```python
from build123d import *

# Parameters (mm, degrees)
ESQUISSE1_R        = 1.5
BOSS_EXTRU_2_DEPTH = 3


with BuildPart() as part:
    # Esquisse1 → Boss.-Extru.2 (new body)
    with BuildSketch(Plane.XY):
        with BuildLine():
            Line((-6, -33.155494421), (-6, -30.155494421))
            Line((-6, -30.155494421), (-7, -30.155494421))
            Line((-7, -30.155494421), (-7, -26.155494421))
            Line((-7, -26.155494421), (-6, -26.155494421))
            Line((-6, -26.155494421), (-6, -12.649110641))
            ThreePointArc((-6, -12.649110641), (-6.653410863, -12.317959405), (-7.288606081, -11.953084179))
            ThreePointArc((-7.288606081, -11.953084179), (-8.912631465, -10.307392628), (-9.031496673, -7.998360322))
            ThreePointArc((-9.031496673, -7.998360322), (-9.309773091, -5.375), (-11.442531564, -3.822325392))
            ThreePointArc((-11.442531564, -3.822325392), (-13.054716827, -2.946828253), (-13.935938611, -1.337764944))
            ThreePointArc((-13.935938611, -1.337764944), (-12.367555464, 6.560760004), (-6.707371512, 12.288660114))
            ThreePointArc((-6.707371512, 12.288660114), (-4.47014813, 12.872261577), (-2.411034891, 11.820685714))
            ThreePointArc((-2.411034891, 11.820685714), (0, 10.75), (2.411034891, 11.820685714))
            ThreePointArc((2.411034891, 11.820685714), (3.975330286, 12.779130538), (5.80943088, 12.737759334))
            ThreePointArc((5.80943088, 12.737759334), (11.865562564, 7.430237213), (13.995977593, -0.335575935))
            ThreePointArc((13.995977593, -0.335575935), (13.382779595, -2.564868949), (11.442531564, -3.822325392))
            ThreePointArc((11.442531564, -3.822325392), (9.309773091, -5.375), (9.031496673, -7.998360322))
            ThreePointArc((9.031496673, -7.998360322), (9.079386541, -9.832302285), (8.126507731, -11.399994391))
            ThreePointArc((8.126507731, -11.399994391), (7.090812931, -12.071469338), (6, -12.649110641))
            Line((6, -12.649110641), (6, -26.155494421))
            Line((6, -26.155494421), (7, -26.155494421))
            Line((7, -26.155494421), (7, -30.155494421))
            Line((7, -30.155494421), (6, -30.155494421))
            Line((6, -30.155494421), (6, -33.155494421))
            Line((6, -33.155494421), (10, -33.155494421))
            Line((10, -33.155494421), (10, -16.155494421))
            ThreePointArc((10, -16.155494421), (0, 19), (-10, -16.155494421))
            Line((-10, -16.155494421), (-10, -33.155494421))
            Line((-10, -33.155494421), (-6, -33.155494421))
        make_face()
        with Locations((0, 14)):
            Circle(ESQUISSE1_R, mode=Mode.SUBTRACT)
        with Locations((12.124355653, -7)):
            Circle(ESQUISSE1_R, mode=Mode.SUBTRACT)
        with Locations((-12.124355653, -7)):
            Circle(ESQUISSE1_R, mode=Mode.SUBTRACT)
    extrude(amount=BOSS_EXTRU_2_DEPTH)


solid = part.part
```
The model under review builds one solid part; all positions refer to its coordinate system, in mm. A direction names the side the tool comes from. Coordinates: 2 decimals unless noted, no trailing zeros. Order: outer loops, then holes, each group sorted by start corner. A loop starts at its lowest first (then second) coordinate and runs counter-clockwise, first axis right, second up. Notation, with made-up numbers: (-6, 50) -> (18, 50) arc R19 cw to (18, 68) -> close; hole circle Ø10 at (-14.75, 25.5). An arc over 180 degrees is marked (long way). Answer in a Markdown table with one row per item. Add a question column.
Item 1: Machinability: for faces 5 (the flat face through (-10, -5, 3)), 6 (the flat face through (-7, -28, 1)), 7 (the flat face through (6, -32, 1)), 8 (the flat face through (-10, -25, 1)), 9 (the flat face through (-10, -5, 0)), which of the approach directions +Z, -Z, +X, -X, +Y, -Y give a long, thin tool a straight path to every point of the face, cutting with its end or side? Answer none if there is none.
Item 2: Clearance check with flat-ended pins moving along their axes: pin 1 (1 mm diameter, centred on y = -11, z = 1, fed in from -X); pin 2 (1.1 mm diameter, centred on x = 6.5, z = 2, fed in from +Y); pin 3 (0.9 mm diameter, centred on y = -17, z = 1.5, fed in from -X). State where each tip first meets the part, or that it passes through.
Item 3: Mouldability with a two-part tool opening along X and no side actions: class faces 1 (the flat face through (6.5, -26.155, 1.5)), 2 (the flat face through (7, -28, 1)), 3 (the flat face through (-8, -33.155, 1)), 4 (the flat face through (10, -25, 1)) as +X half, -X half, draft (parallel to the pull), parting line (faces both ways), or undercut.
Item 4: To check wall thickness, follow probe 1 along X at (y, z) = (-22, 2.45); probe 2 along Y at (x, z) = (12.5, 0.2); probe 3 along Y at (x, z) = (0, 2.35). State the ranges of each line that lie inside material, in increasing order.
Item 5: We need section C-C on y = -7. Write out the cut boundary in (x, z), plus the area to 3 significant figures.
Item 6: We need section A-A on x = 0. Write out the cut boundary in (y, z).
Item 7: We need section D-D on z = 2.1. Give the number of separate pieces and of enclosed holes in the cut face, plus the area to 3 significant figures.
Item 8: We need section B-B on y = 14. Write out the cut boundary in (x, z), plus the area to 3 significant figures.
Final values:
| question | item | result |
|---|---|---|
| 1 | face 5 | +Z, +X, -X, +Y, -Y |
| 1 | face 6 | +Z, -Z |
| 1 | face 7 | +Z, -Z, -Y |
| 1 | face 8 | +Z, -Z, -X, -Y |
| 1 | face 9 | -Z, +X, -X, +Y, -Y |
| 2 | pin 1 | stops at x = -15.84 |
| 2 | pin 2 | stops at y = 18.04 |
| 2 | pin 3 | stops at x = -10 |
| 3 | face 1 | undercut |
| 3 | face 2 | undercut |
| 3 | face 3 | draft |
| 3 | face 4 | +X half |
| 4 | probe 1 | x = -10 to -6, 6 to 10 |
| 4 | probe 2 | y = -14.31 to -8.45, -5.55 to -3.39, 6.3 to 14.31 |
| 4 | probe 3 | y = 10.75 to 12.5, 15.5 to 19 |
| 5 | outline | (-17.66, 0) -> (-13.62, 0) -> (-13.62, 3) -> (-17.66, 3) -> close; (-10.62, 0) -> (-8.87, 0) -> (-8.87, 3) -> (-10.62, 3) -> close; (8.87, 0) -> (10.62, 0) -> (10.62, 3) -> (8.87, 3) -> close; (13.62, 0) -> (17.66, 0) -> (17.66, 3) -> (13.62, 3) -> close |
| 5 | area | 34.7 mm2 |
| 6 | outline | (10.75, 0) -> (12.5, 0) -> (12.5, 3) -> (10.75, 3) -> close; (15.5, 0) -> (19, 0) -> (19, 3) -> (15.5, 3) -> close |
| 7 | separate pieces | 1 |
| 7 | enclosed holes | 3 |
| 7 | area | 611 mm2 |
| 8 | outline | (-12.85, 0) -> (-1.5, 0) -> (-1.5, 3) -> (-12.85, 3) -> close; (1.5, 0) -> (12.85, 0) -> (12.85, 3) -> (1.5, 3) -> close |
| 8 | area | 68.1 mm2 |
